Part model, mm, in its own coordinate system. Face numbers are marked on the shaded views. A direction names the side the tool comes from. Round coordinates to 2 decimals unless told otherwise and drop trailing zeros. Order: outer loops, then holes, each group sorted by start corner. A loop starts at its lowest first (then second) coordinate and runs counter-clockwise, first axis right, second up. Notation, with made-up numbers: M -8,-30.5 L 13,-30.5 A29 cw 13,3.5 Z; hole C 6.5,33.25 d11. An arc over 180 degrees is marked long. One line per question, with ' | ' between items.
from build123d import *

# Parameters (mm, degrees)
F0_R     = 6.5
F1_DEPTH = 2.25
F1_TAPER = -45
F2_DEPTH = 0.75
F4_R     = 2
F5_DEPTH = 6


with BuildPart() as f1:
    # F0 (on Top) → F1 (new body)
    with BuildSketch(Plane.XY):
        Circle(F0_R)
    extrude(amount=F1_DEPTH, taper=F1_TAPER)

    # F2 (add): a face of the model
    f2_faces = [f1.faces().sort_by_distance(p)[0] for p in [
        (0, 0, 2.25),
    ]]
    extrude(f2_faces, amount=F2_DEPTH)

    # F3: F1 across plane


with BuildPart() as f1_1:
    add(f1.part)
    add(f1.part.mirror(Plane.XY))

    # F4 (on face) → F5 (cut, through all)
    with BuildSketch(Plane.XY.offset(3)):
        Circle(F4_R)
    extrude(amount=-F5_DEPTH, mode=Mode.SUBTRACT)


solid = f1_1.part
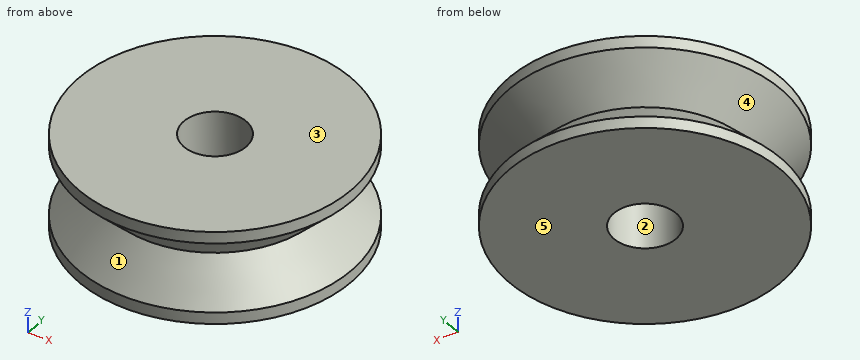
1) Drop flat-ended pins along their axis: pin 1 (3.5 mm diameter, centred on x = 0, y = 0, fed in from -Z); pin 2 (1 mm diameter, centred on y = 2, z = 0, fed in from -X); pin 3 (2 mm diameter, centred on y = 3.5, z = 1.5, fed in from -X). Give the stop position or say it passes through.
The answers:
pin 1: passes through | pin 2: stops at x = -6.73 | pin 3: stops at x = -8.28
2) Probe line 1 (Y direction, x = 0, z = 1.6); line 2 (Z direction, x = 5.25, y = -6.25); line 3 (Y direction, x = 1.5, z = 1.95). List the from-to ranges inside material, lowest first. Write a range as [from, to].
The answers:
line 1: y = [-8.1, -2], [2, 8.1] | line 2: z = [-3, -1.66], [1.66, 3] | line 3: y = [-8.32, -1.32], [1.32, 8.32]
3) Saw through at B-B (z = 0.35). List the corners of the cut face in (x, y), plus the area to 3 significant figures.
The answers:
outline: C 0,0 d13.7; hole C 0,0 d4 | area: 135 mm²
4) Saw through at A-A (x = 0). List the corners of the cut face in (y, z).
The answers:
outline: M -8.75,-3 L -2,-3 L -2,3 L -8.75,3 L -8.75,2.25 L -6.5,0 L -8.75,-2.25 Z; M 2,-3 L 8.75,-3 L 8.75,-2.25 L 6.5,0 L 8.75,2.25 L 8.75,3 L 2,3 Z
5) Saw through at C-C (z = -2). List the corners of the cut face in (x, y), plus the area to 3 significant figures.
The answers:
outline: C 0,0 d17; hole C 0,0 d4 | area: 214 mm²
6) Which spindle directions (+Z, -Z, +X, -X, +Y, -Y) get a long thin tool onto all of the face, cutting with end or side? Do the marked faces 1 and 2. Say none if no direction does.
The answers:
face 1: none | face 2: +Z, -Z
7) Two-plate mould, pull along Z, no slides. Class the marked faces 3, 4 and 5: released by +Z, released by -Z, zero draft, split by the parting line, or undercut.
The answers:
face 3: released by +Z | face 4: undercut | face 5: released by -Z
